from build123d import *

# Parameters (mm, degrees)
BOSS_EXTRUDE1_DEPTH  = 3
M4_CLEARANCE_HOLE1_D = 4.5
SKETCH5_R            = 2
CUT_EXTRUDE1_DEPTH   = 20
SKETCH8_R            = 3
CUT_EXTRUDE3_DEPTH   = 25.596747752


with BuildPart() as part:
    # Sketch2 → Boss-Extrude1 (new, symmetric)
    with BuildSketch(Plane.XY):
        with BuildLine():
            Line((13, 0), (13, -20))
            Line((13, -20), (7, -20))
            Line((7, -20), (7, -10.95445115))
            ThreePointArc((7, -10.95445115), (-11.401754251, 6.244997998), (13, 0))
        make_face()
    extrude(amount=BOSS_EXTRUDE1_DEPTH, both=True)

    # M4 Clearance Hole1 (through all)
    with Locations(Plane.XY.offset(3)):
        with Locations((0, 0)):
            Hole(M4_CLEARANCE_HOLE1_D / 2)

    # Sketch5 → Cut-Extrude1 (cut)
    with BuildSketch(Plane.XZ.offset(20)):
        with Locations(Location((10, 0, 0), (0, 0, 270))):
            Circle(SKETCH5_R)
    extrude(amount=-CUT_EXTRUDE1_DEPTH, mode=Mode.SUBTRACT)

    # Sketch8 → Cut-Extrude3 (cut, through all)
    with BuildSketch(Plane.XY.offset(-3)):
        with Locations((-6.894399988, 5.785088487)):
            Circle(SKETCH8_R)
    extrude(amount=CUT_EXTRUDE3_DEPTH, mode=Mode.SUBTRACT)


solid = part.part
The listing builds one solid part. Answer for the finished solid, in the listing's coordinates (mm). Give positions to 0.01 mm unless a question says otherwise; leave off trailing zeros. Order: outer loops, then holes, each group sorted by start corner. A loop starts at its lowest first (then second) coordinate and runs counter-clockwise, first axis right, second up. Notation, with made-up numbers: (30.5, -26) - (80.5, -26) arc R18 ccw to (80.5, -7) - close; hole circle Ø7 at (9, 43.5). An arc over 180 degrees is marked (long way). Use one line per item in the form item = value.
1) Find section D-D on x = -7.5. Determine the outline of the cut face in (y, z), and give its area (3 significant figures).
Verdict:
outline = (-10.62, -3) - (2.85, -3) - (2.85, 3) - (-10.62, 3) - close; (8.72, -3) - (10.62, -3) - (10.62, 3) - (8.72, 3) - close
area = 92.2 mm^2
2) Find section C-C on z = 1. Determine the outline of the cut face in (x, y).
Verdict:
outline = (7, -20) - (8.27, -20) - (8.27, 0) - (11.73, 0) - (11.73, -20) - (13, -20) - (13, 0) arc R13 ccw (long way) to (7, -10.95) - close; hole circle Ø6 at (-6.89, 5.79); hole circle Ø4.5 at (0, 0)
3) Consider probe 1 along X at (y, z) = (-1, -0.1); probe 2 along X at (y, z) = (8.5, 1.4); probe 3 along X at (y, z) = (6, 2.25). Determine where each line is inside the solid, lowest interval first. Write a range as [from, to].
Verdict:
probe_1 = [-12.96, -2.02], [2.02, 8], [12, 13]
probe_2 = [-9.84, -8.17], [-5.62, 9.84]
probe_3 = [-11.53, -9.89], [-3.9, 11.53]
4) Each of these flat-tipped pins is pushed along its axis until it touches: pin 1 (8 mm diameter, centred on x = -6.89, y = 5.79, fed in from -Z); pin 2 (1 mm diameter, centred on y = -14, z = -2.5, fed in from -X); pin 3 (1.2 mm diameter, centred on x = 10, z = -0.5, fed in from -Y); pin 4 (2.5 mm diameter, centred on x = 10, z = 0, fed in from +Y). Where does it stop, or does it pass through?
Verdict:
pin_1 = -3
pin_2 = 7
pin_3 = 0
pin_4 = 9.61
5) Find section A-A on x = 0. Determine the outline of the cut face in (y, z).
Verdict:
outline = (-13, -3) - (-2.25, -3) - (-2.25, 3) - (-13, 3) - close; (2.25, -3) - (13, -3) - (13, 3) - (2.25, 3) - close
6) The mould has two halves that part along Z. Classify faces 1 (the flat face through (3, -3, 3)), 2 (the flat face through (7, -16, 0)), 3 (the cylindrical face through (12, -10, 0)), 4 (the flat face through (10, 0, 0)): released by +Z, released by -Z, zero draft, split by the parting line, or undercut.
Verdict:
face_1 = released by +Z
face_2 = zero draft
face_3 = undercut
face_4 = undercut
7) Find section B-B on y = -5. Determine the outline of the cut face in (x, z), and give its area (3 significant figures).
Verdict:
outline = (-12, -3) - (13, -3) - (13, 3) - (-12, 3) - close; hole circle Ø4 at (10, 0)
area = 137 mm^2
